Can you work these out from the model? Positions are in its coordinate system, mm. A direction names the side the tool comes from. Coordinates: 2 decimals unless noted, no trailing zeros. Loops run counter-clockwise (first coordinate to the right, second up) from the corner with the lowest first, then second, coordinate; pieces in that order, holes last.
```python
from build123d import *

# Parameters (mm, degrees)
F1_W     = 77.895202
F1_H     = 53.751212
F2_DEPTH = 25.4
F0_R     = 27.177432
F3_DEPTH = 38.1
F4_R     = 5.08
F5_R     = 14.999896
F6_DEPTH = 76.201
F7_SIZE  = 5.08


with BuildPart() as f2:
    # F1 (on Top) → F2 (new body)
    with BuildSketch(Plane.XY):
        with Locations((1.762334, -1.674218)):
            Rectangle(F1_W, F1_H)
    extrude(amount=F2_DEPTH)

    # F0 (on Front) → F3 (join, symmetric)
    with BuildSketch(Plane.XZ):
        Circle(F0_R)
    extrude(amount=F3_DEPTH, both=True)

    # F4
    f4_edges = [f2.edges().sort_by_distance(p)[0] for p in [
        (40.709935, -28.549824, 12.7),
        (40.709935, 25.201388, 12.7),
        (40.709935, -1.674218, 0),
        (40.709935, -1.674218, 25.4),
        (-37.185267, 25.201388, 12.7),
        (-37.185267, -28.549824, 12.7),
        (-37.185267, -1.674218, 0),
        (-37.185267, -1.674218, 25.4),
    ]]
    fillet(f4_edges, radius=F4_R)

    # F5 (on face) → F6 (cut, through all)
    with BuildSketch(Plane.XZ.offset(38.1)):
        Circle(F5_R)
    extrude(amount=-F6_DEPTH, mode=Mode.SUBTRACT)

    # F7
    f7_edges = [f2.edges().sort_by_distance(p)[0] for p in [
        (-14.999896, -38.1, 0),
        (-14.999896, 38.1, 0),
    ]]
    chamfer(f7_edges, length=F7_SIZE)


solid = f2.part
```
(1) I want a section at A-A on x = 0. Write out the boundary of the cut face in (y, z).
Check values:
outline: (-38.1, -27.18) - (38.1, -27.18) - (38.1, -20.08) - (33.02, -15) - (-33.02, -15) - (-38.1, -20.08) - close; (-38.1, 20.08) - (-33.02, 15) - (33.02, 15) - (38.1, 20.08) - (38.1, 27.18) - (-38.1, 27.18) - close
(2) If I drill on probe 1 along Z at (x, y) = (0, 7.5); probe 2 along Z at (x, y) = (12, 13); probe 3 along Z at (x, y) = (-29.5, -10), over which ranges is the centre line in solid material (lowest first)?
Check values:
probe 1: z = -27.18 to -15, 15 to 27.18
probe 2: z = -24.38 to -9, 9 to 25.4
probe 3: z = 0 to 25.4
(3) I want a section at D-D on y = 26.5. Write out the boundary of the cut face in (x, z), then the cut area to 3 significant figures.
Check values:
outline: circle Ø54.35 at (0, 0); hole circle Ø30 at (0, 0)
area: 1,610 mm2
(4) I want a section at C-C on x = -23.5. Write out the boundary of the cut face in (y, z).
Check values:
outline: (-38.1, -13.65) - (38.1, -13.65) - (38.1, 13.65) - (25.2, 13.65) - (25.2, 25.4) - (-28.55, 25.4) - (-28.55, 13.65) - (-38.1, 13.65) - close
(5) Which directions (+Z, -Z, +X, -X, +Y, -Y) give clear straight access to the entire face, cutting with the end or side of a thin tool? Please do faces 1 (the flat face through (22, -1, 25.4)), 2 (the flat face through (-26, -28.55, 15)), 3 (the flat face through (-26, 25.201, 15)).
Check values:
face 1: +Z, +X, +Y, -Y
face 2: +Z, -X, -Y
face 3: +Z, -X, +Y
(6) I want a section at B-B on y = -16. Write out the boundary of the cut face in (x, z).
Check values:
outline: (-37.19, 5.08) arc R5.08 ccw to (-32.11, 0) - (-27.18, 0) arc R27.18 ccw to (27.18, 0) - (35.63, 0) arc R5.08 ccw to (40.71, 5.08) - (40.71, 20.32) arc R5.08 ccw to (35.63, 25.4) - (9.67, 25.4) arc R27.18 ccw to (-9.67, 25.4) - (-32.11, 25.4) arc R5.08 ccw to (-37.19, 20.32) - close; hole circle Ø30 at (0, 0)
(7) I'm going to push flat-ended pins straight in: pin 1 (8 mm diameter, centred on x = 23, y = -9, fed in from +Z); pin 2 (8 mm diameter, centred on y = 16.5, z = -5, fed in from -X); pin 3 (2 mm diameter, centred on x = -14.5, z = -12, fed in from +Y). Where does each tip first touch, or does it pass through?
Check values:
pin 1: stops at z = 25.4
pin 2: stops at x = -27.16
pin 3: stops at y = 37.84
(8) If we mould it in two halves opening along Z, with no side actions, what happens to faces 4 (the flat face through (31, -1, 0)), 5 (the flat face through (28, 25.201, 15)), 6 (the cylindrical face through (39.182, -1.298, 23.951)), 7 (the cylindrical face through (-3.252, -0.462, -14.643))? For each: released by +Z, released by -Z, zero draft, split by the parting line, or undercut.
Check values:
face 4: released by -Z
face 5: zero draft
face 6: released by +Z
face 7: undercut
